from build123d import *

# Parameters (mm, degrees)
CYLINDER_R           = 2.65
CYLINDER_DEPTH       = 21
CYLINDER001_R        = 11.25
CYLINDER001_DEPTH    = 2
BOX_W                = 42.2
BOX_H                = 42.2
BOX_DEPTH            = 24
CHAMFER_SIZE         = 4
CYLINDER002_R        = 1.65
CYLINDER002_DEPTH    = 16.5
POLARPATTERN_COUNT   = 4
BOX001_W             = 17.85
BOX001_H             = 2.1
BOX001_DEPTH         = 5
BODY_PLACEMENT_ANGLE = 90


with BuildPart() as part:
    # Cylinder → Cylinder (join)
    with BuildSketch(Plane.XY):
        Circle(CYLINDER_R)
    extrude(amount=CYLINDER_DEPTH)

    # Cylinder001 → Cylinder001 (join)
    with BuildSketch(Plane(origin=(0, 0, 0), x_dir=(1, 0, 0), z_dir=(0, 0, -1))):
        Circle(CYLINDER001_R)
    extrude(amount=CYLINDER001_DEPTH)

    # Box → Box (join)
    with BuildSketch(Plane(origin=(-21.1, 21.1, -2), x_dir=(1, 0, 0), z_dir=(0, 0, -1))):
        with Locations((21.1, 21.1)):
            Rectangle(BOX_W, BOX_H)
    extrude(amount=BOX_DEPTH)

    # Chamfer
    chamfer_edges = [part.edges().sort_by_distance(p)[0] for p in [
        (-21.1, 21.1, -14),
        (-21.1, -21.1, -14),
        (21.1, -21.1, -14),
        (21.1, 21.1, -14),
    ]]
    chamfer(chamfer_edges, length=CHAMFER_SIZE)

    # Cylinder002 → Cylinder002 (join)
    with BuildSketch(Plane(origin=(-15.5, -15.5, -2), x_dir=(1, 0, 0), z_dir=(0, 0, 1))):
        Circle(CYLINDER002_R)
    cylinder002 = extrude(amount=CYLINDER002_DEPTH)

    # Cone → Cone (revolve)
    with BuildSketch(Plane(origin=(-15.5, -15.5, 14.5), x_dir=(1, 0, 0), z_dir=(0, -1, 0))):
        Polygon((0, 0), (1.65, 0), (3, 1.75), (0, 1.75), align=None)
    cone = revolve(axis=Axis((-15.5, -15.5, 14.5), (0, 0, 1)))

    # PolarPattern: Cylinder002, Cone ×4 about axis
    polarpattern_axis = Axis((0, 0, 0), (0, 0, 1))
    for i in range(1, POLARPATTERN_COUNT):
        add(cylinder002.rotate(polarpattern_axis, i * 360 / POLARPATTERN_COUNT))
        add(cone.rotate(polarpattern_axis, i * 360 / POLARPATTERN_COUNT))

    # Box001 → Box001 (cut)
    with BuildSketch(Plane(origin=(-4, -2.5, 3.15), x_dir=(0, 0, 1), z_dir=(0, 1, 0))):
        with Locations((8.925, 1.05)):
            Rectangle(BOX001_W, BOX001_H)
    extrude(amount=BOX001_DEPTH, mode=Mode.SUBTRACT)


with BuildPart() as part_1:
    # Body placement: moved
    add(part.part.moved(Location((0, 0, 1))).rotate(Axis((0, 0, 1), (0, 0, -1)), BODY_PLACEMENT_ANGLE))


solid = part_1.part
For this review, take the finished solid that the model builds, in its own axes (mm). A direction names the side the tool comes from. Round coordinates to 2 decimals unless told otherwise and drop trailing zeros. Write each loop counter-clockwise with the first axis right and the second up, starting at its lowest first coordinate (ties: lowest second). Pieces come first, ordered by that corner, then holes. Notation, with made-up numbers: M -25,-23 L -21,-23 A7 cw -21,-16 Z; hole C 69,18.5 d9. An arc over 180 degrees is marked long. Write item = value, one per line. Start each with the question number.
(1) We need section A-A (z = 11). Give the boundary of the cut face in (x, y).
(2) For faces 1 (the face through (-19.1, -19.1, -12.8)), 2 (the face through (9.98, -5.19, 0.01)), 3 (the face through (-15.004, 13.926, 7.134)), list the 3-axis set-ups (+Z, -Z, +X, -X, +Y, -Y) from which the entire face can be reached by the end or side of a thin tool; tool diameter is ignored.
(3) For line 1 along Z through (x, y) = (-12, -5.5); line 2 along Z through (x, y) = (2, 3); line 3 along Z through (x, y) = (15.5, -13), list the stretches that pass through material, from the lowest coordinate up.
(4) Clearance check with flat-ended pins moving along their axes: pin 1 Ø1.5 at (x, z) = (-12, 4) entering from +Y; pin 2 Ø1.8 at (x, z) = (-1, 13.5) entering from +Y; pin 3 Ø3 at (x, y) = (16, 14.5) entering from +Z; pin 4 Ø2 at (y, z) = (9.5, 0.5) entering from +X. State where each tip first meets the part, or that it passes through.
(5) We need section D-D (x = 15.5). Give the boundary of the cut face in (y, z).
(6) We need section C-C (z = -15.5). Give the boundary of the cut face in (x, y).
(7) We need section B-B (y = 9). Give the boundary of the cut face in (x, z).
(8) The part is to be moulded in two halves that separate along X. For faces 4 (the face through (-21.1, 0, -13)), 5 (the face through (-1.01, -2.45, 11.35)), 6 (the face through (15, -16, 17.25)), 7 (the face through (15.004, -13.926, 7.134)), say which applies: +X half, -X half, draft (parallel to the pull), parting line (faces both ways), or undercut.
Results found:
q1.outline = C -15.5,-15.5 d3.3; C -15.5,15.5 d3.3; M -1.85,1.9 A2.65 ccw long 1.85,1.9 Z; C 15.5,-15.5 d3.3; C 15.5,15.5 d3.3
q2.face_1 = +Z, -Z, -X, -Y
q2.face_2 = +Z
q2.face_3 = none
q3.line_1 = -25 to -1
q3.line_2 = -25 to 1
q3.line_3 = -25 to -1, 16.6 to 17.25
q4.pin_1 = through
q4.pin_2 = 1.9
q4.pin_3 = 17.25
q4.pin_4 = 7.37
q5.outline = M -21.1,-25 L 21.1,-25 L 21.1,-1 L 17.15,-1 L 17.15,15.5 L 18.5,17.25 L 12.5,17.25 L 13.85,15.5 L 13.85,-1 L -13.85,-1 L -13.85,15.5 L -12.5,17.25 L -18.5,17.25 L -17.15,15.5 L -17.15,-1 L -21.1,-1 Z
q6.outline = M -21.1,-17.1 L -17.1,-21.1 L 17.1,-21.1 L 21.1,-17.1 L 21.1,17.1 L 17.1,21.1 L -17.1,21.1 L -21.1,17.1 Z
q7.outline = M -21.1,-25 L 21.1,-25 L 21.1,-1 L 6.75,-1 L 6.75,1 L -6.75,1 L -6.75,-1 L -21.1,-1 Z
q8.face_4 = -X half
q8.face_5 = parting line
q8.face_6 = draft
q8.face_7 = undercut
